```python
from build123d import *

# Parameters (mm, degrees)
EXTRUDE_1_DEPTH          = 125
M4X0_7_1_D               = 3.3
M4X0_7_1_DEPTH           = 11.5
M4X0_7_1_TIP             = 0.991420021
M4X0_7_1_ON_FACE_2_D     = 3.3
M4X0_7_1_ON_FACE_2_DEPTH = 11.5
M4X0_7_1_ON_FACE_2_TIP   = 0.991420021


with BuildPart() as part:
    # ｽｹｯﾁ1 → ﾎﾞｽ - 押し出し1 (new body)
    with BuildSketch(Plane.XY):
        Polygon((0, 0), (15, 0), (15, 2), (2, 2), (2, 15), (0, 15), align=None)
    extrude(amount=EXTRUDE_1_DEPTH)

    # M4x0.7 ねじ穴1
    with Locations(Plane(origin=(7.5, 0, 10), x_dir=(0, 0, -1), z_dir=(0, -1, 0))):
        with Locations((0, 0), (-100, 0)):
            Hole(M4X0_7_1_D / 2, depth=M4X0_7_1_DEPTH)
            with Locations((0, 0, -(M4X0_7_1_DEPTH + M4X0_7_1_TIP / 2))):  # 118° drill point
                Cone(0, M4X0_7_1_D / 2, M4X0_7_1_TIP, mode=Mode.SUBTRACT)

    # M4x0.7 ねじ穴1 on face 2
    with Locations(Plane(origin=(0, 7.5, 110), x_dir=(0, 0, -1), z_dir=(-1, 0, 0))):
        with Locations((0, 0), (100, 0)):
            Hole(M4X0_7_1_ON_FACE_2_D / 2, depth=M4X0_7_1_ON_FACE_2_DEPTH)
            with Locations((0, 0, -(M4X0_7_1_ON_FACE_2_DEPTH + M4X0_7_1_ON_FACE_2_TIP / 2))):  # 118° drill point
                Cone(0, M4X0_7_1_ON_FACE_2_D / 2, M4X0_7_1_ON_FACE_2_TIP, mode=Mode.SUBTRACT)


solid = part.part
```
Work out the finished part from the listing and answer in its coordinate system (mm). A direction names the side the tool comes from. Round coordinates to 2 decimals unless told otherwise and drop trailing zeros. Loops run counter-clockwise (first coordinate to the right, second up) from the corner with the lowest first, then second, coordinate; pieces in that order, holes last.
(1) The part is cut by section C-C, the plane y = 11.25. Give the vertices of the cut face in (x, z).
Computed values:
outline: (0, 0) - (2, 0) - (2, 125) - (0, 125) - close
(2) Each of these flat-tipped pins is pushed along its axis until it touches: P1, Ø4, axis at x = 10.5, z = 48, coming from the -Y side; P2, Ø1, axis at y = 4.5, z = 24, coming from the +X side; P3, Ø5.5, axis at x = 7.5, z = 110, coming from the +Y side; P4, Ø3, axis at y = 7.5, z = 110, coming from the +X side. Where does it stop, or does it pass through?
Computed values:
P1: stops at y = 0
P2: stops at x = 2
P3: stops at y = 2
P4: passes through
(3) The part is cut by section D-D, the plane z = 58. Give the vertices of the cut face in (x, y).
Computed values:
outline: (0, 0) - (15, 0) - (15, 2) - (2, 2) - (2, 15) - (0, 15) - close
(4) Find the intervals of material crossed by L1, parallel to Z at x = 0.55, y = 7.5; L2, parallel to X at y = 1.2, z = 10, in increasing order.
Computed values:
L1: z = 0 to 8.35, 11.65 to 108.35, 111.65 to 125
L2: x = 0 to 5.85, 9.15 to 15
(5) The part is cut by section A-A, the plane z = 110. Give the vertices of the cut face in (x, y), and give its area (3 significant figures).
Computed values:
outline: (0, 0) - (5.85, 0) - (5.85, 2) - (2, 2) - (2, 5.85) - (0, 5.85) - close; (0, 9.15) - (2, 9.15) - (2, 15) - (0, 15) - close; (9.15, 0) - (15, 0) - (15, 2) - (9.15, 2) - close
area: 42.8 mm2
(6) The mould has two halves that part along Y. Classify faces 1 (the flat face through (0, 8, 62)), 2 (the cylindrical face through (1.014, 6.385, 108.784)), 3 (the flat face through (1, 15, 62)): pulls with the +Y half, pulls with the -Y half, needs draft (parallel to the pull), parting line crosses it, or undercut.
Computed values:
face 1: needs draft
face 2: undercut
face 3: pulls with the +Y half
(7) The part is cut by section B-B, the plane x = 7.5. Give the vertices of the cut face in (y, z).
Computed values:
outline: (0, 0) - (2, 0) - (2, 8.35) - (0, 8.35) - close; (0, 11.65) - (2, 11.65) - (2, 108.35) - (0, 108.35) - close; (0, 111.65) - (2, 111.65) - (2, 125) - (0, 125) - close
(8) For faces 4 (the flat face through (1, 5, 0)), 5 (the flat face through (9, 2, 62)), determine the directions among +Z, -Z, +X, -X, +Y, -Y from which every point of the face is accessible in a straight line to the end or side of a thin tool.
Computed values:
face 4: -Z, +X, -X, +Y, -Y
face 5: +Z, -Z, +X, +Y
